Check sheet for the modelled part. Datum: model origin and axes. Units: mm. Face numbers are marked on the shaded views. A direction names the side the tool comes from. Give positions to 0.01 mm unless a question says otherwise; leave off trailing zeros. Loops run counter-clockwise (first coordinate to the right, second up) from the corner with the lowest first, then second, coordinate; pieces in that order, holes last. Notation, with made-up numbers: (79.25, 30.25) - (110.25, 30.25) arc R10 cw to (110.25, 42.25) - close; hole circle Ø2 at (-29.75, 42). An arc over 180 degrees is marked (long way). Answer in a Markdown table with one row per item. Add a question column.
(1) Thickness scan on L1, parallel to Z at x = -83, y = 1.3; L2, parallel to Y at x = -80, z = 13.25; L3, parallel to X at y = 3.25, z = 11.5. Record the ranges inside material, lowest first.
(2) Set-up check for the marked faces 1 and 2: record each of +Z, -Z, +X, -X, +Y, -Y from which the full face is reachable in a straight line by a thin tool's end or side.
(3) Go/stop test with flat-tipped pins: P1, Ø5, axis at x = -83, z = 71.2, coming from the +Y side; P2, Ø1.5, axis at x = -48, z = 54.5, coming from the +Y side; P3, Ø1.5, axis at y = 4, z = 37.5, coming from the -X side; P4, Ø4, axis at x = -20, z = 86.2, coming from the -Y side. Record where each tip stops, or that it passes through.
(4) Sectioned sample at A-A on x = -46.75. Enter the section's corners in (y, z).
(5) Sectioned sample at B-B on z = 13. Enter the section's corners in (x, y), then the cut area to 3 significant figures.
(6) Sectioned sample at C-C on z = 90.5. Enter the section's corners in (x, y).
(7) Sectioned sample at D-D on z = 61.5. Enter the section's corners in (x, y).
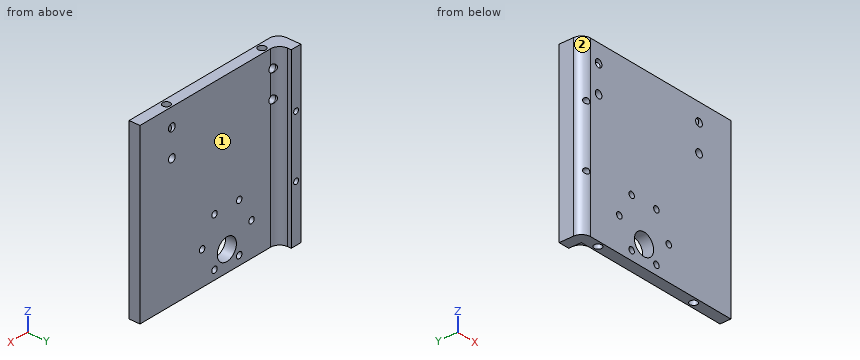
from build123d import *

# Parameters (mm, degrees)
SKETCH1_W           = 93
SKETCH1_H           = 96.2019
SKETCH1_R           = 6
SKETCH1_R_2         = 1.7
SKETCH1_R_3         = 2.1
BOSS_EXTRUDE1_DEPTH = 6
BOSS_EXTRUDE2_START = -6
SKETCH2_W           = 6
SKETCH2_H           = 96.2019
SKETCH2_R           = 1.5
BOSS_EXTRUDE2_DEPTH = 7
SKETCH2_3_R         = 1.5
CUT_EXTRUDE2_DEPTH  = 135.435135153
SKETCH3_R           = 2.1
CUT_EXTRUDE3_DEPTH  = 18
CUT_EXTRUDE4_START  = -78.2019
SKETCH3_2_R         = 2.1
CUT_EXTRUDE4_DEPTH  = 18
FILLET1_R           = 5


with BuildPart() as part:
    # Sketch1 → Boss-Extrude1 (new body)
    with BuildSketch(Plane(origin=(0, 0, 0), x_dir=(-1, 0, 0), z_dir=(0, 1, 0))):
        with Locations((46.5, 48.10095)):
            Rectangle(SKETCH1_W, SKETCH1_H)
        with Locations(Location((54.5, 11.5, 0), (0, 0, 90))):
            Circle(SKETCH1_R, mode=Mode.SUBTRACT)
        with Locations(Location((39, 18.5, 0), (0, 0, 90))):
            Circle(SKETCH1_R_2, mode=Mode.SUBTRACT)
        with Locations(Location((46.75, 31.923393759, 0), (0, 0, 90))):
            Circle(SKETCH1_R_2, mode=Mode.SUBTRACT)
        with Locations(Location((62.25, 31.923393759, 0), (0, 0, 90))):
            Circle(SKETCH1_R_2, mode=Mode.SUBTRACT)
        with Locations(Location((70, 18.5, 0), (0, 0, 90))):
            Circle(SKETCH1_R_2, mode=Mode.SUBTRACT)
        with Locations(Location((62.25, 5.076606241, 0), (0, 0, 90))):
            Circle(SKETCH1_R_2, mode=Mode.SUBTRACT)
        with Locations(Location((46.75, 5.076606241, 0), (0, 0, 90))):
            Circle(SKETCH1_R_2, mode=Mode.SUBTRACT)
        with Locations(Location((20, 86.2019, 0), (0, 0, 90))):
            Circle(SKETCH1_R_3, mode=Mode.SUBTRACT)
        with Locations(Location((83, 86.2019, 0), (0, 0, 90))):
            Circle(SKETCH1_R_3, mode=Mode.SUBTRACT)
        with Locations(Location((83, 71.2019, 0), (0, 0, 90))):
            Circle(SKETCH1_R_3, mode=Mode.SUBTRACT)
        with Locations(Location((20, 71.2019, 0), (0, 0, 90))):
            Circle(SKETCH1_R_3, mode=Mode.SUBTRACT)
    extrude(amount=BOSS_EXTRUDE1_DEPTH)

    # Sketch2 → Boss-Extrude2 (add)
    with BuildSketch(Plane(origin=(0, 0, 0), x_dir=(-1, 0, 0), z_dir=(0, -1, 0)).offset(BOSS_EXTRUDE2_START)):
        with Locations((90, -48.10095)):
            Rectangle(SKETCH2_W, SKETCH2_H)
        with Locations(Location((90, -65.10095, 0), (0, 0, 90))):
            Circle(SKETCH2_R, mode=Mode.SUBTRACT)
        with Locations(Location((90, -31.10095, 0), (0, 0, 90))):
            Circle(SKETCH2_R, mode=Mode.SUBTRACT)
    extrude(amount=-BOSS_EXTRUDE2_DEPTH)

    # Sketch2<3> → Cut-Extrude2 (cut, through all)
    with BuildSketch(Plane(origin=(0, 0, 0), x_dir=(-1, 0, 0), z_dir=(0, -1, 0))):
        with Locations(Location((90, -31.10095, 0), (0, 0, 90))):
            Circle(SKETCH2_3_R)
        with Locations(Location((90, -65.10095, 0), (0, 0, 90))):
            Circle(SKETCH2_3_R)
    extrude(amount=-CUT_EXTRUDE2_DEPTH, mode=Mode.SUBTRACT)

    # Sketch3 → Cut-Extrude3 (cut)
    with BuildSketch(Plane(origin=(0, 0, 0), x_dir=(1, 0, 0), z_dir=(0, 0, -1))):
        with Locations(Location((-80, -3, 0), (0, 0, 180))):
            Circle(SKETCH3_R)
        with Locations(Location((-20, -3, 0), (0, 0, 180))):
            Circle(SKETCH3_R)
    extrude(amount=-CUT_EXTRUDE3_DEPTH, mode=Mode.SUBTRACT)

    # Sketch3<2> → Cut-Extrude4 (cut)
    with BuildSketch(Plane(origin=(0, 0, 0), x_dir=(1, 0, 0), z_dir=(0, 0, -1)).offset(CUT_EXTRUDE4_START)):
        with Locations(Location((-80, -3, 0), (0, 0, 180))):
            Circle(SKETCH3_2_R)
        with Locations(Location((-20, -3, 0), (0, 0, 180))):
            Circle(SKETCH3_2_R)
    extrude(amount=-CUT_EXTRUDE4_DEPTH, mode=Mode.SUBTRACT)

    # Fillet1
    # the kernel refuses this fillet: 5 mm, written as the material it adds along each edge
    with BuildSketch(Plane(origin=(-87, 6, 96.2019), x_dir=(1, 0, 0), z_dir=(0, 0, -1))) as fillet1_piece_1_section:
        with BuildLine():
            CenterArc((FILLET1_R, -FILLET1_R), FILLET1_R, 90, 90)
            Line((0, -FILLET1_R), (0, 0))
            Line((0, 0), (FILLET1_R, 0))
        make_face()
    fillet1_piece_1 = extrude(amount=96.2019, mode=Mode.PRIVATE)
    fillet1_piece_1 = fillet1_piece_1 - Plane(origin=(-83, 7.144811059, 71.2019), x_dir=(0, 0, 1), z_dir=(0, -1, 0)) * Cylinder(2.1, 213, mode=Mode.PRIVATE)
    fillet1_piece_1 = fillet1_piece_1 - Plane(origin=(-83, 7.144811059, 86.2019), x_dir=(0, 0, 1), z_dir=(0, -1, 0)) * Cylinder(2.1, 213, mode=Mode.PRIVATE)
    add(fillet1_piece_1)
    # the kernel refuses this fillet: 5 mm, written as the material it takes off along each edge
    with BuildSketch(Plane(origin=(-93, 0, -12.5), x_dir=(1, 0, 0), z_dir=(0, 0, 1))) as fillet1_2_piece_1:
        with BuildLine():
            CenterArc((FILLET1_R, FILLET1_R), FILLET1_R, 180, 90)
            Line((0, FILLET1_R), (0, 0))
            Line((0, 0), (FILLET1_R, 0))
        make_face()
    extrude(amount=121.2019, mode=Mode.SUBTRACT)


solid = part.part
Reply:
| question | item | result |
|---|---|---|
| 1 | L1 | 0 to 69.1, 73.3 to 84.1, 88.3 to 96.2 |
| 1 | L2 | 0 to 0.9, 5.1 to 6 |
| 1 | L3 | -92.68 to -82.09, -77.91 to -60.5, -48.5 to -22.09, -17.91 to 0 |
| 2 | face 1 | +Z, -Z, +X, +Y |
| 2 | face 2 | +Z, -Z, -X, -Y |
| 3 | P1 | y = 7.43 |
| 3 | P2 | y = 6 |
| 3 | P3 | x = -92.99 |
| 3 | P4 | through |
| 4 | outline | (0, 0) - (6, 0) - (6, 3.38) - (0, 3.38) - close; (0, 6.78) - (6, 6.78) - (6, 30.22) - (0, 30.22) - close; (0, 33.62) - (6, 33.62) - (6, 96.2) - (0, 96.2) - close |
| 5 | outline | (-93, 5) arc R5 ccw to (-88, 0) - (-60.31, 0) - (-60.31, 6) - (-82, 6) arc R5 cw to (-87, 11) - (-87, 13) - (-93, 13) - close; (-48.69, 0) - (0, 0) - (0, 6) - (-48.69, 6) - close; hole circle Ø4.2 at (-80, 3); hole circle Ø4.2 at (-20, 3) |
| 5 | area | 503 mm^2 |
| 6 | outline | (-93, 5) arc R5 ccw to (-88, 0) - (0, 0) - (0, 6) - (-82, 6) arc R5 cw to (-87, 11) - (-87, 13) - (-93, 13) - close; hole circle Ø4.2 at (-80, 3); hole circle Ø4.2 at (-20, 3) |
| 7 | outline | (-93, 5) arc R5 ccw to (-88, 0) - (0, 0) - (0, 6) - (-82, 6) arc R5 cw to (-87, 11) - (-87, 13) - (-93, 13) - close |
